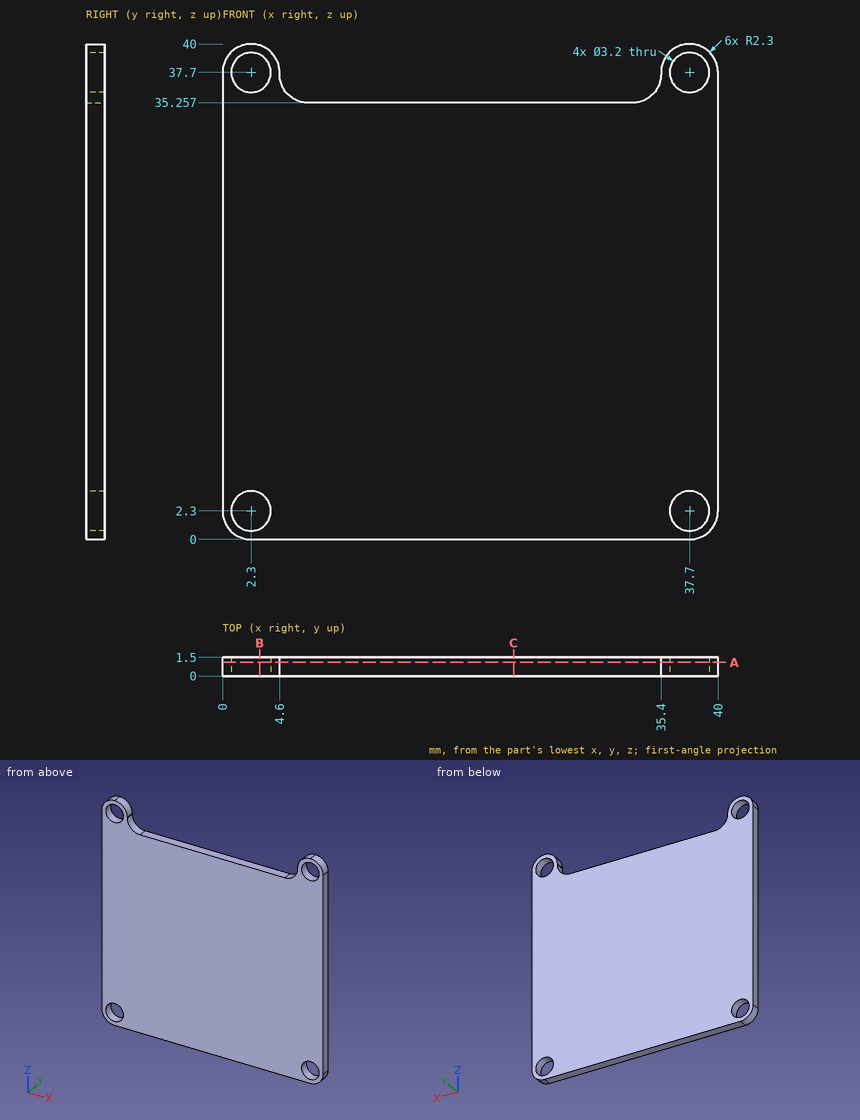
Source: three-view drawing plus pictorial views. Frame: mm from the lowest corner of the part. Give positions to 0.01 mm unless a question says otherwise; leave off trailing zeros. Order: outer loops, then holes, each group sorted by start corner. A loop starts at its lowest first (then second) coordinate and runs counter-clockwise, first axis right, second up. Notation, with made-up numbers: M 1,14.25 L 21,14.25 A11 cw 21,34.25 Z; hole C 29.25,28.25 d10. An arc over 180 degrees is marked long. Return JSON: item names as keys, results as strings.
Item 1: First-contact query: P1, Ø2.5, axis at x = 2.3, z = 2.3, coming from the -Y side. Flat tip, straight axial feed; report the tip coordinate or a pass-through.
Solutions:
{"P1": "through"}
Item 2: Cut plane B-B (x = 3). Return loops of the section in (y, z).
Solutions:
{"outline": "M 0,0 L 1.5,0 L 1.5,0.86 L 0,0.86 Z; M 0,3.74 L 1.5,3.74 L 1.5,36.26 L 0,36.26 Z; M 0,39.14 L 1.5,39.14 L 1.5,39.89 L 0,39.89 Z"}
Item 3: Cut plane C-C (x = 23.5). Return loops of the section in (y, z).
Solutions:
{"outline": "M 0,0 L 1.5,0 L 1.5,35.26 L 0,35.26 Z"}
Item 4: Ray query, probe 1 along X at (y, z) = (0.5, 37.7); probe 2 along Z at (x, y) = (37.7, 0.7); probe 3 along Z at (x, y) = (3, 0.85). Return the intervals inside material, ascending.
Solutions:
{"probe 1": "0 to 0.7, 3.9 to 4.6, 35.4 to 36.1, 39.3 to 40", "probe 2": "0 to 0.7, 3.9 to 36.1, 39.3 to 40", "probe 3": "0 to 0.86, 3.74 to 36.26, 39.14 to 39.89"}
Item 5: Cut plane A-A (y = 1.1). Return loops of the section in (x, z), then the cut area to 3 significant figures.
Solutions:
{"outline": "M 0,2.3 A2.3 ccw 2.3,0 L 37.7,0 A2.3 ccw 40,2.3 L 40,37.7 A2.3 ccw 35.4,37.7 L 35.4,37.56 A2.3 cw 33.1,35.26 L 6.9,35.26 A2.3 cw 4.6,37.56 L 4.6,37.7 A2.3 ccw 0,37.7 Z; hole C 2.3,2.3 d3.2; hole C 2.3,37.7 d3.2; hole C 37.7,2.3 d3.2; hole C 37.7,37.7 d3.2", "area": "1,420 mm^2"}
